from build123d import *

# Parameters (mm, degrees)
F0_W     = 67
F0_H     = 118.5
F1_DEPTH = 2
F3_DEPTH = 2


with BuildPart() as f1:
    # F0 (on Front) → F1 (new body)
    with BuildSketch(Plane.XZ):
        with Locations((33.5, 59.25)):
            Rectangle(F0_W, F0_H)
    extrude(amount=F1_DEPTH)

    # F2 (on face) → F3 (join)
    with BuildSketch(Plane.XY.offset(118.5)):
        with BuildLine():
            Line((2.143183, 0), (64.856817, 0))
            ThreePointArc((64.856817, 0), (33.5, 28.5), (2.143183, 0))
        make_face()
        with BuildLine():
            Line((2.015877, -2), (64.984123, -2))
            ThreePointArc((64.984123, -2), (64.936379, -0.998987), (64.856817, 0))
            Line((64.856817, 0), (2.143183, 0))
            ThreePointArc((2.143183, 0), (2.063621, -0.998987), (2.015877, -2))
        make_face()
    extrude(amount=-F3_DEPTH)


solid = f1.part
The model under review builds one solid part; all positions refer to its coordinate system, in mm. A direction names the side the tool comes from. Round coordinates to 2 decimals unless told otherwise and drop trailing zeros. Order: outer loops, then holes, each group sorted by start corner. A loop starts at its lowest first (then second) coordinate and runs counter-clockwise, first axis right, second up. Notation, with made-up numbers: (25, 32.25) -> (49, 32.25) arc R22 ccw to (49, 47.25) -> close; hole circle Ø2 at (-38.75, 36.5). An arc over 180 degrees is marked (long way). Write item = value, one per line. Start each with the question number.
Item 1: Consider section C-C on y = 2. Write out the cut boundary in (x, z).
Item 2: For line 1 along Y through (x, z) = (20, 96.5); line 2 along Z through (x, y) = (23, 19.5), list the stretches that pass through material, from the lowest coordinate up.
Item 3: Consider section B-B on x = 20.5. Write out the cut boundary in (y, z).
Item 4: Consider section A-A on z = 42. Write out the cut boundary in (x, y).
Item 5: Consider section D-D on x = 54.5. Write out the cut boundary in (y, z), plus the area to 3 significant figures.
Item 6: Clearance check with flat-ended pins moving along their axes: pin 1 Ø1 at (x, z) = (37, 96) entering from +Y; pin 2 Ø3 at (x, y) = (15, 11.5) entering from -Z. State where each tip first meets the part, or that it passes through.
Item 7: For faces 1 (the face through (33, 11, 116.5)), 2 (the face through (33, -2, 60)), list the 3-axis set-ups (+Z, -Z, +X, -X, +Y, -Y) from which the entire face can be reached by the end or side of a thin tool; tool diameter is ignored.
Conclusion:
q1.outline = (2.4, 116.5) -> (64.6, 116.5) -> (64.6, 118.5) -> (2.4, 118.5) -> close
q2.line_1 = -2 to 0
q2.line_2 = 116.5 to 118.5
q3.outline = (-2, 0) -> (0, 0) -> (0, 116.5) -> (25.69, 116.5) -> (25.69, 118.5) -> (-2, 118.5) -> close
q4.outline = (0, -2) -> (67, -2) -> (67, 0) -> (0, 0) -> close
q5.outline = (-2, 0) -> (0, 0) -> (0, 116.5) -> (20.48, 116.5) -> (20.48, 118.5) -> (-2, 118.5) -> close
q5.area = 278 mm2
q6.pin_1 = 0
q6.pin_2 = 116.5
q7.face_1 = -Z, +X, -X, +Y
q7.face_2 = +Z, -Z, +X, -X, -Y
